Check sheet for the drawn part. Datum: minimum x, y, z corner. Units: mm. A direction names the side the tool comes from. Round coordinates to 2 decimals unless told otherwise and drop trailing zeros. Order: outer loops, then holes, each group sorted by start corner. A loop starts at its lowest first (then second) coordinate and runs counter-clockwise, first axis right, second up. Notation, with made-up numbers: (-37, 75.5) -> (-4, 75.5) arc R16 ccw to (-4, 91.5) -> close; hole circle Ø4 at (-30, 31). An arc over 180 degrees is marked (long way). Answer as a JSON object with one key per item and string values. Group by question number.
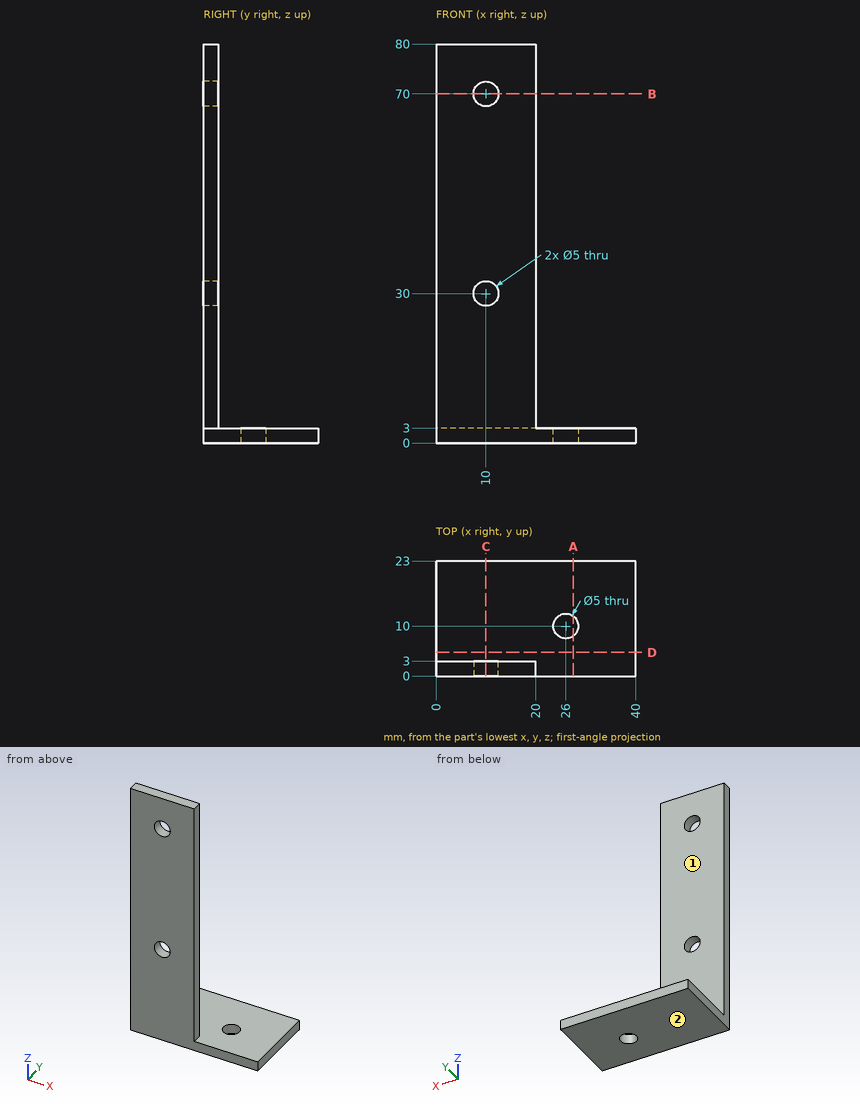
Item 1: Set-up check for the marked faces 1 and 2: record each of +Z, -Z, +X, -X, +Y, -Y from which the full face is reachable in a straight line by a thin tool's end or side.
Item 2: Sectioned sample at C-C, the plane x = 10. Enter the section's corners in (y, z), then the cut area to 3 significant figures.
Item 3: Sectioned sample at D-D, the plane y = 4.75. Enter the section's corners in (x, z).
Item 4: Thickness scan on L1, parallel to Z at x = 10, y = 1.6; L2, parallel to X at y = 0.7, z = 70; L3, parallel to Z at x = 30.5, y = 10.75. Record the ranges inside material, lowest first.
Item 5: Depth check by flat-ended pin: pin 1 Ø4.5 at (x, y) = (26, 10) entering from +Z; pin 2 Ø7 at (x, y) = (29.5, 16) entering from +Z; pin 3 Ø10 at (x, z) = (12, 50) entering from +Y; pin 4 Ø0.9 at (y, z) = (1, 37) entering from +X. Enter the tip coordinate at first touch or a pass-through.
Item 6: Sectioned sample at A-A, the plane x = 27.5. Enter the section's corners in (y, z), then the cut area to 3 significant figures.
Item 7: Sectioned sample at B-B, the plane z = 70. Enter the section's corners in (x, y).
Result:
{
 "1": {"face 1": "+Z, +X, -X, +Y", "face 2": "-Z, +X, -X, +Y, -Y"},
 "2": {"outline": "(0, 0) -> (23, 0) -> (23, 3) -> (3, 3) -> (3, 27.5) -> (0, 27.5) -> close; (0, 32.5) -> (3, 32.5) -> (3, 67.5) -> (0, 67.5) -> close; (0, 72.5) -> (3, 72.5) -> (3, 80) -> (0, 80) -> close", "area": "270 mm2"},
 "3": {"outline": "(0, 0) -> (40, 0) -> (40, 3) -> (0, 3) -> close"},
 "4": {"L1": "z = 0 to 27.5, 32.5 to 67.5, 72.5 to 80", "L2": "x = 0 to 7.5, 12.5 to 20", "L3": "z = 0 to 3"},
 "5": {"pin 1": "passes through", "pin 2": "stops at z = 3", "pin 3": "stops at y = 3", "pin 4": "stops at x = 20"},
 "6": {"outline": "(0, 0) -> (8, 0) -> (8, 3) -> (0, 3) -> close; (12, 0) -> (23, 0) -> (23, 3) -> (12, 3) -> close", "area": "57.0 mm2"},
 "7": {"outline": "(0, 0) -> (7.5, 0) -> (7.5, 3) -> (0, 3) -> close; (12.5, 0) -> (20, 0) -> (20, 3) -> (12.5, 3) -> close"}
}
